from build123d import *

# Parameters (mm, degrees)
F0_R     = 25.4
F1_DEPTH = 6.35
F0_W     = 139.7
F0_H     = 76.2
F0_R_2   = 28.575
F2_DEPTH = 44.45
F3_D     = 13.096875
F5_D     = 9.8044
F5_DEPTH = 38.101
F6_D     = 9.8044


with BuildPart() as f1:
    # F0 (on Top) → F1 (new body)
    with BuildSketch(Plane.XY):
        Circle(F0_R)
    extrude(amount=F1_DEPTH)



with BuildPart() as f1b:
    # F0 (on Top) → F1, piece 2 (new body)
    with BuildSketch(Plane.XY):
        Rectangle(F0_W, F0_H)
        Circle(F0_R_2, mode=Mode.SUBTRACT)
    extrude(amount=F1_DEPTH)


with BuildPart() as f1_1:
    add(f1.part)

    add(f1b.part)  # F2 merges F1b
    # F0 (on Top) → F2 (join)
    with BuildSketch(Plane.XY):
        Circle(F0_R_2)
        Circle(F0_R, mode=Mode.SUBTRACT)
    extrude(amount=F2_DEPTH)

    # F3 (through all)
    with Locations(Plane(origin=(0, 0, 0), x_dir=(1, 0, 0), z_dir=(0, 0, -1))):
        with Locations((-50.8, -19.05), (50.8, -19.05), (50.8, 19.05), (-50.8, 19.05)):
            Hole(F3_D / 2)

    # F5 (through all, one way)
    with BuildSketch(Plane(origin=(0, 0, 0), x_dir=(1, 0, 0), z_dir=(0, 1, 0))):
        with Locations((0, -25.4)):
            Circle(F5_D / 2)
    extrude(amount=-F5_DEPTH, mode=Mode.SUBTRACT)

    # F6 (through all)
    with Locations(Plane.XZ):
        with Locations((0, 25.4)):
            Hole(F6_D / 2)


solid = f1_1.part
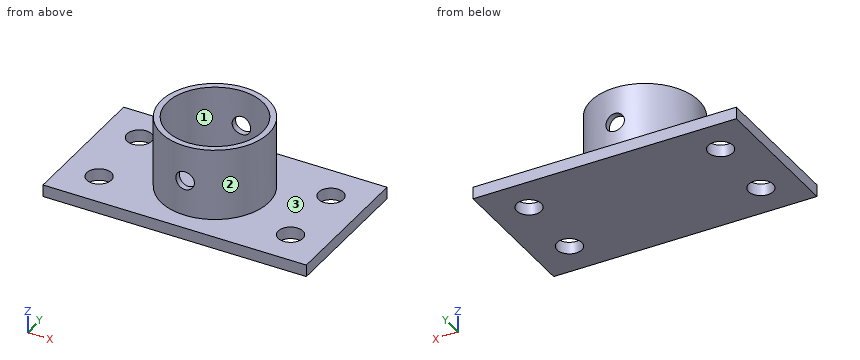
Model file for the job. Use its own axes, mm. Face numbers are marked on the shaded views. Give positions to 0.01 mm unless a question says otherwise; leave off trailing zeros. Loops run counter-clockwise (first coordinate to the right, second up) from the corner with the lowest first, then second, coordinate; pieces in that order, holes last.
1) Saw through at B-B (y = 0). Write the cut outline in (x, z) (3 decimals).
2) Wall check: line 1 (X direction, y = 19.05, z = 3.5); line 2 (Y direction, x = -50.8, z = 4.5); line 3 (Y direction, x = -49.5, z = 4). Give the ranges that are in metal, low to high.
3) Saw through at C-C (z = 25.4). Write the cut outline in (x, y) (3 decimals), plus the area to 3 significant figures.
4) Saw through at D-D (y = -19.05). Write the cut outline in (x, z), plus the area to 3 significant figures.
5) Saw through at A-A (x = 0). Write the cut outline in (y, z) (3 decimals).
6) Pull direction X, two halves, no side cores. Call the marked faces 1, 2 and 3: +X half, -X half, draft (parallel to the pull), parting line (faces both ways), or undercut.
7) Flat gauge pins, fed straight in: pin 1 Ø21 at (x, y) = (50.8, -19.05) entering from -Z; pin 2 Ø10.5 at (x, y) = (-50.8, 19.05) entering from +Z; pin 3 Ø3 at (y, z) = (15, 16.5) entering from -X; pin 4 Ø6 at (y, z) = (-22.5, 11.5) entering from -X. Where does each tip first touch, or does it go through?
Answer block:
1. outline: (-69.85, 0) - (69.85, 0) - (69.85, 6.35) - (28.575, 6.35) - (28.575, 44.45) - (25.4, 44.45) - (25.4, 6.35) - (-25.4, 6.35) - (-25.4, 44.45) - (-28.575, 44.45) - (-28.575, 6.35) - (-69.85, 6.35) - close
2. line 1: x = -69.85 to -57.35, -44.25 to 44.25, 57.35 to 69.85
2. line 2: y = -38.1 to -25.6, -12.5 to 12.5, 25.6 to 38.1
2. line 3: y = -38.1 to -25.47, -12.63 to 12.63, 25.47 to 38.1
3. outline: (-4.902, -28.151) - (-4.902, -24.922) arc R25.4 cw to (-4.902, 24.922) - (-4.902, 28.151) arc R28.575 ccw to start; (4.902, -28.151) arc R28.575 ccw to (4.902, 28.151) - (4.902, 24.922) arc R25.4 cw to (4.902, -24.922) - close
3. area: 476 mm2
4. outline: (-69.85, 0) - (-57.35, 0) - (-57.35, 6.35) - (-69.85, 6.35) - close; (-44.25, 0) - (44.25, 0) - (44.25, 6.35) - (21.3, 6.35) - (21.3, 44.45) - (16.8, 44.45) - (16.8, 6.35) - (-16.8, 6.35) - (-16.8, 44.45) - (-21.3, 44.45) - (-21.3, 6.35) - (-44.25, 6.35) - close; (57.35, 0) - (69.85, 0) - (69.85, 6.35) - (57.35, 6.35) - close
4. area: 1,060 mm2
5. outline: (-38.1, 0) - (38.1, 0) - (38.1, 6.35) - (28.575, 6.35) - (28.575, 20.498) - (25.4, 20.498) - (25.4, 6.35) - (-25.4, 6.35) - (-25.4, 20.498) - (-28.575, 20.498) - (-28.575, 6.35) - (-38.1, 6.35) - close; (-28.575, 30.302) - (-25.4, 30.302) - (-25.4, 44.45) - (-28.575, 44.45) - close; (25.4, 30.302) - (28.575, 30.302) - (28.575, 44.45) - (25.4, 44.45) - close
6. face 1: undercut
6. face 2: parting line
6. face 3: draft
7. pin 1: stops at z = 0
7. pin 2: passes through
7. pin 3: stops at x = -25.18
7. pin 4: stops at x = -20.89
